Build history of the part. All positions in model axes, mm. Face numbers are marked on the shaded views. A direction names the side the tool comes from. Give positions to 0.01 mm unless a question says otherwise; leave off trailing zeros. Order: outer loops, then holes, each group sorted by start corner. A loop starts at its lowest first (then second) coordinate and runs counter-clockwise, first axis right, second up. Notation, with made-up numbers: M -13,-11.5 L 46,-11.5 A27 cw 46,8.5 Z; hole C -2,86.5 d4. An arc over 180 degrees is marked long. Answer as CSV lines item,"result".
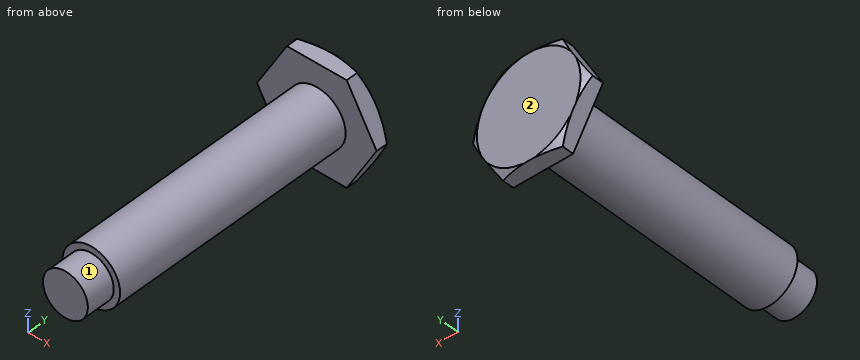
from build123d import *

# Parameters (mm, degrees)
BOSS_EXTRUDE1_DEPTH = 1.4
SKETCH2_OUTSIDE_W   = 18.618
SKETCH2_OUTSIDE_H   = 17.226
SKETCH2_OUTSIDE_R   = 4.5
CUT_EXTRUDE1_DEPTH  = 1
CUT_EXTRUDE1_TAPER  = 60
SKETCH3_R           = 2.5
BOSS_EXTRUDE2_DEPTH = 24.3
SKETCH4_OUTSIDE_W   = 18.218
SKETCH4_OUTSIDE_H   = 16.826
SKETCH4_OUTSIDE_R   = 1.95
CUT_EXTRUDE2_DEPTH  = 2.5


with BuildPart() as part:
    # Sketch1 → Boss-Extrude1 (new body)
    with BuildSketch(Plane(origin=(0, 0, 0), x_dir=(1, 0, 0), z_dir=(0, 1, 0))):
        Polygon((5.195, 0), (2.5975, 4.499001973), (-2.5975, 4.499001973), (-5.195, 0), (-2.5975, -4.499001973), (2.5975, -4.499001973), align=None)
    extrude(amount=BOSS_EXTRUDE1_DEPTH)

    # Sketch2 outside → Cut-Extrude1 (cut)
    with BuildSketch(Plane(origin=(0, 1.4, 0), x_dir=(1, 0, 0), z_dir=(0, 1, 0))):
        Rectangle(SKETCH2_OUTSIDE_W, SKETCH2_OUTSIDE_H)
        Circle(SKETCH2_OUTSIDE_R, mode=Mode.SUBTRACT)
    extrude(amount=-CUT_EXTRUDE1_DEPTH, taper=CUT_EXTRUDE1_TAPER, mode=Mode.SUBTRACT)

    # Sketch3 → Boss-Extrude2 (add)
    with BuildSketch(Plane.XZ):
        Circle(SKETCH3_R)
    extrude(amount=BOSS_EXTRUDE2_DEPTH)

    # Sketch4 outside → Cut-Extrude2 (cut)
    with BuildSketch(Plane.XZ.offset(24.3)):
        Rectangle(SKETCH4_OUTSIDE_W, SKETCH4_OUTSIDE_H)
        Circle(SKETCH4_OUTSIDE_R, mode=Mode.SUBTRACT)
    extrude(amount=-CUT_EXTRUDE2_DEPTH, mode=Mode.SUBTRACT)


solid = part.part
Item 1: Band-saw the part on A-A (y = -7.75). Give the cut face in (x, z).
Geometry says:
outline,"C 0,0 d5"
Item 2: Probe line 1 along Y through (x, z) = (-3.5, 0); line 2 along X through (y, z) = (-12.75, 0); line 3 along Z through (x, y) = (-1.25, -9.5). List the from-to ranges inside material, lowest first. Write a range as from..to.
Geometry says:
line 1,"y = 0..1.4"
line 2,"x = -2.5..2.5"
line 3,"z = -2.17..2.17"
Item 3: 3-axis set-ups, long thin cutter, end or side, ignore diameter. For the marked faces 1 and 2: which of +Z, -Z, +X, -X, +Y, -Y reach the whole face in a straight line?
Geometry says:
face 1,"-Y"
face 2,"+Z, -Z, +X, -X, +Y"
Item 4: Drop flat-ended pins along their axis: pin 1 (1.5 mm diameter, centred on y = -16.5, z = 2.5, fed in from -X); pin 2 (3 mm diameter, centred on y = -10, z = -3.5, fed in from -X). Give the stop position or say it passes through.
Geometry says:
pin 1,"stops at x = -1.79"
pin 2,"stops at x = -1.5"
